Input: part model. Units: mm. Frame: model coordinates. Face numbers are marked on the shaded views. A direction names the side the tool comes from. Give positions to 0.01 mm unless a question says otherwise; leave off trailing zeros. Loops run counter-clockwise (first coordinate to the right, second up) from the corner with the lowest first, then second, coordinate; pieces in that order, holes last. Notation, with made-up numbers: (87.25, 35) - (107.25, 35) arc R28 ccw to (107.25, 59) - close; hole circle Ø2 at (-18, 80.25). An arc over 180 degrees is marked (long way). One line per question, with ' | ' between items. Start each with the question number.
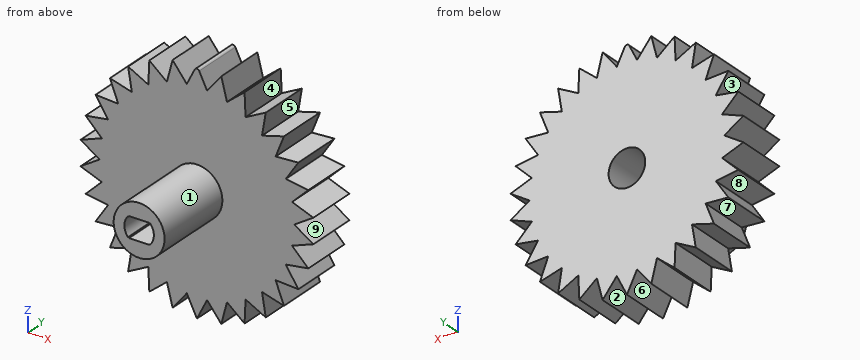
Autodesk Inventor part; units mm, degrees
ref_plane "YZ Plane" through (0, 0, 0) normal (1, 0, 0) x (0, 1, 0)
ref_plane "XZ Plane" through (0, 0, 0) normal (0, 1, 0) x (-1, 0, 0)
ref_plane "XY Plane" through (0, 0, 0) normal (0, 0, 1) x (1, 0, 0)
sketch "Sketch1" plane through (0, 0, 0) normal (0, 1, 0) x (-1, 0, 0)
  line L0 (-2, 0) -> (2, 0)
  line L1 (-2, 0) -> (-2, 1)
  line L2 (-2, 1) -> (0, 0)
  line L3 (0, 0) -> (2, 1)
  line L4 (0, 0) -> (0, 19)
  line L5 (0, 19) -> (2, 19)
  line L6 (-2, 19) -> (0, 19)
  line L7 (0, 19) -> (0, 23)
  line L8 (0, 23) -> (-2, 19)
  line L9 (2, 19) -> (0, 23)
  line L10 (2, 0) -> (2, 19)
  line L11 (-2, 19) -> (-2, 0)
  point P0 (0, 41)
  dimension "d6" = 1
  dimension "d10" = 19
  dimension "d11" = 4
extrude "Extrusion1" add sketch "Sketch1" along normal blind 26 contours L3 L10 L0 | L4 L5 L10 L3 | L2 L11 L6 L4 | L7 L9 L5 | L6 L8 L7
pattern_circular "Circular Pattern1" count 30 over 360 about axis through (0, 0, 0) along (0, 1, 0) of "Extrusion1"
fillet "Fillet1" radius 0.5 1 edges at (0, 13, 23)
sketch "Sketch2" plane through (0, 26, 0) normal (0, 1, 0) x (1, 0, 0)
  circle A0 centre (0, 0) radius 1.5
  circle A1 centre (0, 0) radius 2.8
  line L0 (0, 0) -> (0, 1.9)
  line L1 (0, 1.9) -> (0, -1.9)
  line L2 (0, -1.9) -> (-2.0567, -1.9)
  line L3 (0, -1.9) -> (2.0567, -1.9)
  line L4 (0, 1.9) -> (2.0567, 1.9)
  line L5 (0, 1.9) -> (-2.0567, 1.9)
  circle A2 centre (0, 0) radius 3.6
  line L6 (0, 0) -> (0, 0.7)
  line L7 (0, 0) -> (0, -0.7)
  circle A3 centre (0, 0) radius 2.9
  line L8 (0, 0.7) -> (-2.8142, 0.7)
  line L9 (0, -0.7) -> (-2.8142, -0.7)
  line L10 (0, -0.7) -> (2.8142, -0.7)
  line L11 (0, 0.7) -> (2.8142, 0.7)
  circle A4 centre (0, 0) radius 5
  circle A5 centre (0, 0) radius 15
  circle A6 centre (0, 0) radius 30.1844
  line L12 (-2.0567, 1.9) -> (-2.1909, 1.9)
  line L13 (-2.1909, -1.9) -> (-2.0567, -1.9)
  line L14 (2.0567, -1.9) -> (2.1909, -1.9)
  line L15 (2.0567, 1.9) -> (2.1909, 1.9)
  line L16 (-1.0864, -1.9) -> (-1.0864, -2)
  line L17 (-1.0864, 1.9) -> (-1.0864, 2)
  line L18 (-1.0864, 2) -> (-2.1, 2)
  line L19 (-1.0864, 2) -> (2.1, 2)
  line L20 (-2.1, -2) -> (-1.0864, -2)
  line L21 (-1.0864, -2) -> (2.1, -2)
  circle A7 centre (0, 0) radius 3
  point P0 (1.9596, -2)
  point P1 (-1.9596, -2)
  point P2 (1.9596, 2)
  point P3 (-1.9596, 2)
  dimension "d30" = 5.8
  dimension "d13" = 3
  dimension "d19" = 5.6
  dimension "d20" = 1.9
  dimension "d21" = 3.8
  dimension "d27" = 7.2
  dimension "d28" = 0.7
  dimension "d29" = 0.7
  dimension "d37" = 10
  dimension "d38" = 30
  dimension "d43" = 0.1
  dimension "d44" = 0.1
  dimension "d47" = 6
extrude "Extrusion2" cut sketch "Sketch2" against normal blind 7.5 contours A0 L10 L1 L0 L11 | A0 L11 A1 L10 | L11 L0 A0 | A0 L0 L4 A1 L11 | L10 A1 L3 L1 A0 | A0 L1 L10 | L0 L8 A0 | A0 L8 A1 L5 L0 | L0 L1 L9 A0 L8 | L11 A3 L10 A1 | A1 L15 A3 L11 | L1 L2 A1 L9 A0 | A0 L9 L1 | L10 A3 L14 A1 | A0 L9 A1 L8 | L5 L17 L19 A1 L4 | A1 L19 A3 L15 | L3 A1 L21 L16 L2 | L14 A3 L21 A1 | L8 A3 L12 A1 | A1 L9 A3 L8 | L5 A1 L18 L17 | L19 L18 A1 | A1 L18 A3 L19 | A1 L13 A3 L9 | L16 L20 A1 L2 | L21 A3 L20 A1 | A1 L20 L21 | L12 A3 L18 A1 | A1 L20 A3 L13 | A2 | A7
pattern_circular "Circular Pattern2" [suppressed]
extrude "Extrusion4" cut sketch "Sketch2" against normal blind 8.5 from surface at -7.5 contours A0 L10 L1 L0 L11 | A0 L11 A1 L10 | L11 L0 A0 | A0 L0 L4 A1 L11 | L10 A1 L3 L1 A0 | A0 L1 L10 | L0 L8 A0 | A0 L8 A1 L5 L0 | L0 L1 L9 A0 L8 | L11 A3 L10 A1 | A1 L15 A3 L11 | L1 L2 A1 L9 A0 | A0 L9 L1 | L10 A3 L14 A1 | A0 L9 A1 L8 | L5 L17 L19 A1 L4 | A1 L19 A3 L15 | L3 A1 L21 L16 L2 | L14 A3 L21 A1 | L8 A3 L12 A1 | A1 L9 A3 L8 | L5 A1 L18 L17 | L19 L18 A1 | A1 L18 A3 L19 | A1 L13 A3 L9 | L16 L20 A1 L2 | L21 A3 L20 A1 | A1 L20 L21 | L12 A3 L18 A1 | A1 L20 A3 L13 | A7
extrude "Extrusion6" cut sketch "Sketch2" along normal blind 10 from surface at -26 contours A0 L10 L1 L0 L11 | A0 L11 A1 L10 | L11 L0 A0 | A0 L0 L4 A1 L11 | L10 A1 L3 L1 A0 | A0 L1 L10 | L0 L8 A0 | A0 L8 A1 L5 L0 | L0 L1 L9 A0 L8 | L11 A3 L10 A1 | A1 L15 A3 L11 | L1 L2 A1 L9 A0 | A0 L9 L1 | L10 A3 L14 A1 | A0 L9 A1 L8 | L5 L17 L19 A1 L4 | L3 A1 L21 L16 L2 | L8 A3 L12 A1 | A1 L9 A3 L8 | L5 A1 L18 L17 | A1 L13 A3 L9 | L16 L20 A1 L2
extrude "Extrusion9" cut sketch "Sketch2" along normal blind 16 from surface at -26 contours A5 | A6
properties part number "motor driven gear straight teeth for potentiometer"
Q1. Line query: L1, parallel to X at y = 14.75, z = 0; L2, parallel to Y at x = 4, z = -8. Output: solid intervals per line, ascending. Write a range as from..to.
Q2. Section C-C, the plane z = -10.5. Output: boundary loops of the cut face in (x, y).
Q3. First-contact query: pin 1 (3 mm diameter, centred on x = -5, z = -17.5, fed in from -Y); pin 2 (1 mm diameter, centred on x = 9.5, y = 16.5, fed in from +Z); pin 3 (2 mm diameter, centred on y = 8, z = -4.5, fed in from -X). Flat tips, straight axial feed; report the tip coordinate or a pass-through.
Q4. Section D-D, the plane x = -7.5. Output: boundary loops of the cut face in (y, z), plus the area to 3 significant figures.
Q5. Section B-B, the plane z = 17.5. Output: boundary loops of the cut face in (x, y), plus the area to 3 significant figures.
Q6. Section A-A, the plane y = 8.5. Output: boundary loops of the cut face in (x, z).
Q7. Draft query along X for the marked faces 6, 7, 8 and 9. Return one class per face: +X half, -X half, draft (parallel to the pull), parting line (faces both ways), or undercut.
Q8. Access query for the marked faces 1, 2, 3, 4 and 5. Directions: +Z, -Z, +X, -X, +Y, -Y. A direction counts if a zero-diameter tool reaches every point of the face in a straight line with its end or side. Return the directions, or none.
Solved:
1) L1: x = -5..-3, 3..5 | L2: y = 16..26
2) outline: (-19.26, 16) - (19.26, 16) - (19.26, 26) - (-19.26, 26) - close
3) pin 1: stops at y = 16 | pin 2: stops at z = 21.01 | pin 3: stops at x = -3.57
4) outline: (16, -19.49) - (26, -19.49) - (26, 19.49) - (16, 19.49) - close | area: 390 mm²
5) outline: (-13.34, 16) - (-11.39, 16) - (-11.39, 26) - (-13.34, 26) - close; (-9.51, 16) - (9.51, 16) - (9.51, 26) - (-9.51, 26) - close; (11.39, 16) - (13.34, 16) - (13.34, 26) - (11.39, 26) - close | area: 229 mm²
6) outline: circle Ø10 at (0, 0); hole (-2.19, -1.9) - (-2.06, -1.9) arc R2.8 ccw to (-1.96, -2) - (1.96, -2) arc R2.8 ccw to (2.06, -1.9) - (2.19, -1.9) arc R2.9 ccw to (2.19, 1.9) - (2.06, 1.9) arc R2.8 ccw to (1.96, 2) - (-1.96, 2) arc R2.8 ccw to (-2.06, 1.9) - (-2.19, 1.9) arc R2.9 ccw to start
7) face 6: undercut | face 7: undercut | face 8: -X half | face 9: +X half
8) face 1: -Y | face 2: -Z, +Y, -Y | face 3: -X, +Y, -Y | face 4: +Z, +Y, -Y | face 5: +Y, -Y
